Part model, mm, in its own coordinate system. A direction names the side the tool comes from. Coordinates: 2 decimals unless noted, no trailing zeros. Order: outer loops, then holes, each group sorted by start corner. A loop starts at its lowest first (then second) coordinate and runs counter-clockwise, first axis right, second up.
Autodesk Fusion 360 part; units mm, degrees
sketch "Sketch1" plane through (0, 0, 0) normal (0, 1, 0) x (1, 0, 0)
  line L0 (0, 0) -> (20.5, 0)
  line L1 (20.5, 0) -> (20.5, -20.5)
  line L2 (20.5, -20.5) -> (0, -20.5)
  line L3 (0, -20.5) -> (0, 0)
  line L4 (0, 0) -> (-4, 0)
  line L5 (-4, 0) -> (-4, 4)
  line L6 (-4, 4) -> (0, 4)
  line L7 (0, 4) -> (0, 0)
  line L8 (-4, 4) -> (24.5, 4)
  line L9 (24.5, 4) -> (24.5, -24.5)
  line L10 (24.5, -24.5) -> (-4, -24.5)
  line L11 (-4, -24.5) -> (-4, 4)
  dimension "d1" = 20.5
  dimension "d2" = 20.5
  dimension "d3" = 4
  dimension "d4" = 4
  dimension "d5" = 28.5
  dimension "d6" = 28.5
extrude "Extrude1" add sketch "Sketch1" along normal blind 20
chamfer "Chamfer1" distance 3 angle 45 5 edges at (24.5, 20, 10.25) (10.25, 20, 24.5) (24.5, 10, 24.5) (24.5, 0, 10.25) (10.25, 0, 24.5)
sketch "Sketch2" plane through (0, 0, -4) normal (0, 0, -1) x (-1, 0, 0)
  line L0 (-24.5, 3) -> (-21.5, 0)
  line L1 (-21.5, 0) -> (4, 0)
  line L2 (4, 0) -> (4, 20)
  line L3 (4, 20) -> (-21.5, 20)
  line L4 (-21.5, 20) -> (-24.5, 17)
  line L5 (-24.5, 17) -> (-24.5, 3)
  line L6 (-24.5, 10) -> (-10.25, 10)
  line L7 (-7.6519, 5.5) -> (-5.0538, 10)
  line L8 (-5.0538, 10) -> (-7.6519, 14.5)
  line L9 (-7.6519, 14.5) -> (-12.8481, 14.5)
  line L10 (-12.8481, 14.5) -> (-15.4462, 10)
  line L11 (-15.4462, 10) -> (-12.8481, 5.5)
  line L12 (-12.8481, 5.5) -> (-7.6519, 5.5)
  point P0 (-10.25, 10)
  dimension "d10" = 14.25
  dimension "d11" = 4.5
extrude "Extrude2" add sketch "Sketch2" along normal blind 4
sketch "Sketch3" plane through (0, 0, -8) normal (0, 0, -1) x (-1, 0, 0)
  line L0 (-7.6519, 5.5) -> (-12.8481, 5.5)
  line L1 (-15.4462, 10) -> (-12.8481, 14.5)
  line L2 (-12.8481, 14.5) -> (-7.6519, 14.5)
  line L3 (-7.6519, 14.5) -> (-5.0538, 10)
  line L4 (-5.0538, 10) -> (-7.6519, 5.5)
  line L5 (-24.5, 17) -> (-24.5, 3)
  line L6 (-24.5, 3) -> (-21.5, 0)
  line L7 (-21.5, 0) -> (4, 0)
  line L8 (4, 0) -> (4, 20)
  line L9 (4, 20) -> (-21.5, 20)
  line L10 (-21.5, 20) -> (-24.5, 17)
  line L11 (-7.6519, 14.5) -> (-5.0538, 14.5)
  line L12 (-5.0538, 14.5) -> (-5.0538, 10)
  line L13 (-15.4462, 10) -> (-15.4462, 14.5)
  line L14 (-15.4462, 14.5) -> (-12.8481, 14.5)
extrude "Extrude3" cut sketch "Sketch3" against normal blind 4 contours L1 L13 L14 | L3 L11 L12
sketch "Sketch4" plane through (0, 0, -8) normal (0, 0, -1) x (-1, 0, 0)
  line L0 (-15.4462, 14.5) -> (-5.0538, 14.5)
  line L1 (-5.0538, 14.5) -> (-5.0538, 10)
  line L2 (-5.0538, 10) -> (-7.6519, 5.5)
  line L3 (-7.6519, 5.5) -> (-12.8481, 5.5)
  line L4 (-12.8481, 5.5) -> (-15.4462, 10)
  line L5 (-15.4462, 10) -> (-15.4462, 14.5)
  line L6 (-24.5, 17) -> (-24.5, 3)
  line L7 (-24.5, 3) -> (-21.5, 0)
  line L8 (-21.5, 0) -> (4, 0)
  line L9 (4, 0) -> (4, 20)
  line L10 (4, 20) -> (-21.5, 20)
  line L11 (-21.5, 20) -> (-24.5, 17)
  line L12 (-10.25, 5.5) -> (-10.25, 10)
  circle A0 centre (-10.25, 10) radius 2
  line L13 (-5.0538, 14.5) -> (-15.4186, 14.5)
  line L14 (-15.4186, 14.5) -> (-15.4186, 5.5)
  line L15 (-15.4186, 5.5) -> (-5.0538, 5.5)
  line L16 (-5.0538, 5.5) -> (-5.0538, 14.5)
  line L17 (7, 22) -> (-27, 22)
  line L18 (-27, 22) -> (-27, -2)
  line L19 (-27, -2) -> (7, -2)
  line L20 (7, -2) -> (7, 22)
  dimension "d16" = 4
extrude "Extrude4" add sketch "Sketch4" along normal blind 5 contours L0 L1 L2 L3 L4 L13 L14 L15 L16 | L4 L14 L15 | L2 L15 L16 | L6 L7 L8 L9 L10 L11
extrude "Extrude5" add 1 faces at (0.0833, 10, -13) along direction (0, 0, -1) blind 1.75
sketch "Sketch5" plane through (-4, 0, 0) normal (-1, 0, 0) x (0, 0, 1)
  line L0 (21.5, 0) -> (24.5, 3)
  line L1 (24.5, 3) -> (24.5, 17)
  line L2 (24.5, 17) -> (21.5, 20)
  line L3 (21.5, 20) -> (-14.75, 20)
  line L4 (-14.75, 20) -> (-14.75, 0)
  line L5 (-14.75, 0) -> (21.5, 0)
  line L6 (-14.75, 20) -> (-4.75, 20)
  line L7 (-4.75, 20) -> (-4.75, 0)
  line L8 (-4.75, 0) -> (-14.75, 0)
  line L9 (-14.75, 0) -> (-14.75, 20)
  dimension "d21" = 10
extrude "Extrude6" add sketch "Sketch5" along normal blind 15 contours L3 L4 L5 L6 L7 L8 L9
sketch "Sketch6" plane through (0, 0, -4.75) normal (0, 0, 1) x (1, 0, 0)
  line L0 (-4, 0) -> (-4, 20)
  line L1 (-4, 20) -> (-19, 20)
  line L2 (-19, 20) -> (-19, 0)
  line L3 (-19, 0) -> (-4, 0)
  line L4 (-19, 10) -> (-11.5, 10)
  circle A0 centre (-11.5, 10) radius 3.5
  dimension "d24" = 7.5
  dimension "d25" = 7
extrude "Extrude7" cut sketch "Sketch6" against normal blind 10 contours A0
sketch "Sketch7" plane through (0, 0, 0) normal (0, -1, 0) x (1, 0, 0)
  line L0 (21.5, -14.75) -> (21.5, 21.5)
  line L1 (21.5, 21.5) -> (-4, 21.5)
  line L2 (-4, 21.5) -> (-4, -4.75)
  line L3 (-4, -4.75) -> (-19, -4.75)
  line L4 (-19, -4.75) -> (-19, -14.75)
  line L5 (-19, -14.75) -> (21.5, -14.75)
  line L6 (0, 20.5) -> (20.5, 20.5)
  line L7 (20.5, 20.5) -> (20.5, 0)
  line L8 (20.5, 0) -> (0, 0)
  line L9 (0, 0) -> (0, 20.5)
  line L10 (-19, -4.75) -> (-19, 10.25)
  circle A0 centre (-19, 10.25) radius 15
  dimension "d28" = 15
extrude "Extrude8" add sketch "Sketch7" against normal blind 20 contours L2 L3 A0
sketch "Sketch8" plane through (0, 0, -14.75) normal (0, 0, -1) x (-1, 0, 0)
  circle A0 centre (11.5, 10) radius 3.5
  line L0 (-15.4462, 14.5) -> (-15.4186, 14.5)
  line L1 (-15.4186, 14.5) -> (-15.4186, 9.9523)
  line L2 (-15.4186, 9.9523) -> (-15.4462, 10)
  line L3 (-15.4462, 10) -> (-15.4462, 14.5)
  circle A1 centre (-10.25, 10) radius 2
  line L4 (-21.5, 20) -> (-24.5, 17)
  line L5 (-24.5, 17) -> (-24.5, 3)
  line L6 (-24.5, 3) -> (-21.5, 0)
  line L7 (-21.5, 0) -> (19, 0)
  line L8 (19, 0) -> (19, 20)
  line L9 (19, 20) -> (-21.5, 20)
  circle A2 centre (11.5, 10) radius 5
  dimension "d31" = 10
extrude "Extrude9" cut sketch "Sketch8" along normal blind -10 and the other way blind 27 contours A2
extrude "Extrude10" cut 1 faces at (-11.9678, 9.7747, -4.75) along direction (0, 0, 1) blind 20
Q1. Cut at A-A on x = 10.25. Write the cut outline in (y, z).
Results list:
outline: (0, -14.75) - (8, -14.75) - (8, -8) - (5.5, -8) - (5.5, -4) - (14.5, -4) - (14.5, -8) - (12, -8) - (12, -14.75) - (20, -14.75) - (20, 0) - (0, 0) - close; (0, 20.5) - (20, 20.5) - (20, 21.5) - (17, 24.5) - (3, 24.5) - (0, 21.5) - close
Q2. Wall check: line 1 along X through (y, z) = (10, -7.75); line 2 along X through (y, z) = (4.5, 15); line 3 along Y through (x, z) = (-11.5, -8.75). Give the ranges that are in metal, low to high.
Results list:
line 1: x = -19 to -15, -8 to 5.05, 15.45 to 24.5
line 2: x = -4 to 0, 20.5 to 24.5
line 3: y = 0 to 6.5, 13.5 to 20
Q3. Cut at C-C on z = 16.5. Write the cut outline in (x, y).
Results list:
outline: (-4, 0) - (0, 0) - (0, 20) - (-4, 20) - close; (20.5, 0) - (21.5, 0) - (24.5, 3) - (24.5, 17) - (21.5, 20) - (20.5, 20) - close
Q4. Cut at B-B on y = 11.25. Count the separate pieces of the cut face and the enclosed holes in it, and give its area (3 significant figures).
Results list:
separate pieces: 3
enclosed holes: 1
area: 740 mm2
Q5. Which spindle directions (+Z, -Z, +X, -X, +Y, -Y) get a long thin tool onto all of the face, cutting with end or side? Do faces 1 (the face through (20.5, 10, 10)), 2 (the face through (5.054, 12, -6)), 3 (the face through (-6.505, 9.78, -2.093)), 4 (the face through (-4, 10, 17)). Say none if no direction does.
Results list:
face 1: +Y, -Y
face 2: none
face 3: +Z
face 4: +Z, -X, +Y, -Y
Q6. Cut at D-D on y = 7. Write the cut outline in (x, z), and give its area (3 significant figures).
Results list:
outline: (-19, -14.75) - (-13.3, -14.75) - (-13.3, -4.75) - (-15.5, -4.75) - (-15.5, -4.34) arc R15 cw to (-19, -4.75) - close; (-9.7, -14.75) - (24.5, -14.75) - (24.5, 21.5) - (21.5, 24.5) - (-4, 24.5) - (-4, 10.25) arc R15 cw to (-7.5, 0.62) - (-7.5, -4.75) - (-9.7, -4.75) - close; hole (0, 0) - (20.5, 0) - (20.5, 20.5) - (0, 20.5) - close; hole (6.79, -8) - (13.71, -8) - (13.71, -4) - (6.79, -4) - close
area: 810 mm2
Q7. Pin check, flat tips, straight feed: pin 1 Ø7 at (y, z) = (6.5, 14) entering from -X; pin 2 Ø2 at (y, z) = (4, 9.5) entering from -X. Stop position of each tip, or through.
Results list:
pin 1: stops at x = -4
pin 2: stops at x = -4.1
Q8. Mould opens along Z. For faces 5 (the face through (-19, 10, -10)), 6 (the face through (-6.81, 7.64, 1.51)), 7 (the face through (6.37, 7.72, -5.97)) say: pulls with the +Z half, pulls with the -Z half, needs draft (parallel to the pull), parting line crosses it, or undercut.
Results list:
face 5: needs draft
face 6: pulls with the +Z half
face 7: undercut
